Design review of the part built by this model. Coordinates are the model's own, in mm. Coordinates: 2 decimals unless noted, no trailing zeros. Loops run counter-clockwise (first coordinate to the right, second up) from the corner with the lowest first, then second, coordinate; pieces in that order, holes last. Notation, with made-up numbers: (-32, 82.5) -> (-27, 82.5) arc R25 ccw to (-27, 121.5) -> close; hole circle Ø6 at (44, 56.5). An arc over 180 degrees is marked (long way). Use one line per item in the form item = value. Start each with the question number.
1. The part is to be moulded in two halves that separate along X. For faces 1 (the face through (91.686, 2.348, 67.898)), 2 (the face through (-138.57, 2.35, -83.59)), 3 (the face through (2, 4.762, -1)), say which applies: released by +X, released by -X, zero draft, split by the parting line, or undercut.
2. Consider section A-A (z = -15.5). State the section outline as (x, y) points.
3. For pin 1 (2.5 mm diameter, centred on x = -1.23, z = 72.24, fed in from +Y), flat-tipped, find the tip position at first contact; note if it passes through.
4. Consider section C-C (y = 1). State how many separate pieces and enclosed holes the cut face has, then the cut area to 3 significant figures.
5. Wall thickness on line 1 (X direction, y = 2.65, z = 30); line 2 (X direction, y = 1.15, z = -30); line 3 (Z direction, x = 68, y = 3.25): over which ranges is each line inside the solid? List them lowest first. Write a range as from..to.
6. Consider section B-B (z = 16). State the section outline as (x, y) points.
from build123d import *

# Parameters (mm, degrees)
BOSS_EXTRUDE1_DEPTH          = 4.7625
SKETCH2_R                    = 1.778
CHASSIS_STANDOFF_DEPTH       = 164.899327351
SKETCH3_R                    = 1.5
VESC_DEPTH                   = 164.899327351
SKETCH13_R                   = 1.778
SKETCH13_W                   = 44.755773095
SKETCH13_H                   = 22.569704292
PCB_DEPTH                    = 164.899327351
SKETCH6_W                    = 90
SKETCH6_H                    = 52
JETSON_DEPTH                 = 164.899327351
SKETCH12_R                   = 1.778
TOP_PLATE_STANDOFF_DEPTH     = 164.899327351
SKETCH14_R                   = 2.413
VELODYNE_INTERFACE_BOX_DEPTH = 164.899327351
SKETCH16_R                   = 6.25
SKETCH16_R_2                 = 4.7625
SWITCH_DEPTH                 = 164.899327351


with BuildPart() as part:
    # Sketch1 → Boss-Extrude1 (new body)
    with BuildSketch(Plane(origin=(0, 0, 0), x_dir=(1, 0, 0), z_dir=(0, 1, 0))):
        with BuildLine():
            Line((-135, 85.09), (135, 85.09))
            ThreePointArc((135, 85.09), (138.535533906, 83.625533906), (140, 80.09))
            Line((140, 80.09), (140, -80.09))
            ThreePointArc((140, -80.09), (138.535533906, -83.625533906), (135, -85.09))
            Line((135, -85.09), (-135, -85.09))
            ThreePointArc((-135, -85.09), (-138.535533906, -83.625533906), (-140, -80.09))
            Line((-140, -80.09), (-140, 80.09))
            ThreePointArc((-140, 80.09), (-138.535533906, 83.625533906), (-135, 85.09))
        make_face()
    extrude(amount=BOSS_EXTRUDE1_DEPTH)

    # Sketch2 → chassis standoff (cut, through all)
    with BuildSketch(Plane(origin=(0, 0, 0), x_dir=(1, 0, 0), z_dir=(0, 1, 0))):
        with Locations(Location((68, 58, 0), (0, 0, 90))):
            Circle(SKETCH2_R)
        with Locations(Location((68, -58, 0), (0, 0, 90))):
            Circle(SKETCH2_R)
        with Locations(Location((-122, 30, 0), (0, 0, 90))):
            Circle(SKETCH2_R)
        with Locations(Location((-122, -30, 0), (0, 0, 90))):
            Circle(SKETCH2_R)
    extrude(amount=CHASSIS_STANDOFF_DEPTH, mode=Mode.SUBTRACT)

    # Sketch3 → vesc (cut, through all)
    with BuildSketch(Plane(origin=(0, 0, 0), x_dir=(1, 0, 0), z_dir=(0, 1, 0))):
        with Locations(Location((57.771213393, -50.24032748, 0), (0, 0, 90))):
            Circle(SKETCH3_R)
        with Locations(Location((57.771213393, -61.74032748, 0), (0, 0, 90))):
            Circle(SKETCH3_R)
        with Locations(Location((-1.228786607, -39.74032748, 0), (0, 0, 90))):
            Circle(SKETCH3_R)
        with Locations(Location((-1.228786607, -72.24032748, 0), (0, 0, 90))):
            Circle(SKETCH3_R)
    extrude(amount=VESC_DEPTH, mode=Mode.SUBTRACT)

    # Sketch13 → pcb (cut, through all)
    with BuildSketch(Plane(origin=(0, 0, 0), x_dir=(1, 0, 0), z_dir=(0, 1, 0))):
        with Locations(Location((-97.170021332, -4.946954695, 0), (0, 0, 90))):
            Circle(SKETCH13_R)
        with Locations(Location((-17.170021332, -4.946954695, 0), (0, 0, 90))):
            Circle(SKETCH13_R)
        with Locations(Location((-17.170021332, -79.946954695, 0), (0, 0, 90))):
            Circle(SKETCH13_R)
        with Locations(Location((-97.170021332, -79.946954695, 0), (0, 0, 90))):
            Circle(SKETCH13_R)
        with Locations((-36.456414677, -19.201465216)):
            Rectangle(SKETCH13_W, SKETCH13_H)
    extrude(amount=PCB_DEPTH, mode=Mode.SUBTRACT)

    # Sketch6 → jetson (cut, through all)
    with BuildSketch(Plane(origin=(0, 0, 0), x_dir=(1, 0, 0), z_dir=(0, 1, 0))):
        with Locations((-62.08, 28.74)):
            Rectangle(SKETCH6_W, SKETCH6_H)
    extrude(amount=JETSON_DEPTH, mode=Mode.SUBTRACT)

    # Sketch12 → top plate standoff (cut, through all)
    with BuildSketch(Plane(origin=(0, 0, 0), x_dir=(1, 0, 0), z_dir=(0, 1, 0))):
        with Locations(Location((-129.82, 78.74, 0), (0, 0, 90))):
            Circle(SKETCH12_R)
        with Locations(Location((-106.98, -78.74, 0), (0, 0, 90))):
            Circle(SKETCH12_R)
        with Locations(Location((25.1, 78.74, 0), (0, 0, 90))):
            Circle(SKETCH12_R)
        with Locations(Location((25.1, -78.74, 0), (0, 0, 90))):
            Circle(SKETCH12_R)
    extrude(amount=TOP_PLATE_STANDOFF_DEPTH, mode=Mode.SUBTRACT)

    # Sketch14 → velodyne interface box (cut, through all)
    with BuildSketch(Plane(origin=(0, 0, 0), x_dir=(1, 0, 0), z_dir=(0, 1, 0))):
        with Locations(Location((89.981111903, 47.625, 0), (0, 0, 90))):
            Circle(SKETCH14_R)
        with Locations(Location((89.981111903, -47.625, 0), (0, 0, 90))):
            Circle(SKETCH14_R)
    extrude(amount=VELODYNE_INTERFACE_BOX_DEPTH, mode=Mode.SUBTRACT)

    # Sketch16 → switch (cut, through all)
    with BuildSketch(Plane(origin=(0, 0, 0), x_dir=(1, 0, 0), z_dir=(0, 1, 0))):
        with Locations(Location((86.14110244, -70.782450254, 0), (0, 0, 90))):
            Circle(SKETCH16_R)
        with Locations(Location((109.644443051, -70.782450254, 0), (0, 0, 90))):
            Circle(SKETCH16_R_2)
    extrude(amount=SWITCH_DEPTH, mode=Mode.SUBTRACT)


solid = part.part
Geometry check:
q1.face_1 = undercut
q1.face_2 = released by -X
q1.face_3 = zero draft
q2.outline = (-140, 0) -> (-107.08, 0) -> (-107.08, 4.76) -> (-140, 4.76) -> close; (-17.08, 0) -> (140, 0) -> (140, 4.76) -> (-17.08, 4.76) -> close
q3.pin_1 = through
q4.separate_pieces = 1
q4.enclosed_holes = 22
q4.area = 41,600 mm²
q5.line_1 = -140..-123.78, -120.22..-58.83, -14.08..140
q5.line_2 = -140..-123.78, -120.22..-107.08, -17.08..140
q5.line_3 = -85.09..-59.78, -56.22..56.22, 59.78..85.09
q6.outline = (-140, 0) -> (-58.83, 0) -> (-58.83, 4.76) -> (-140, 4.76) -> close; (-14.08, 0) -> (140, 0) -> (140, 4.76) -> (-14.08, 4.76) -> close
